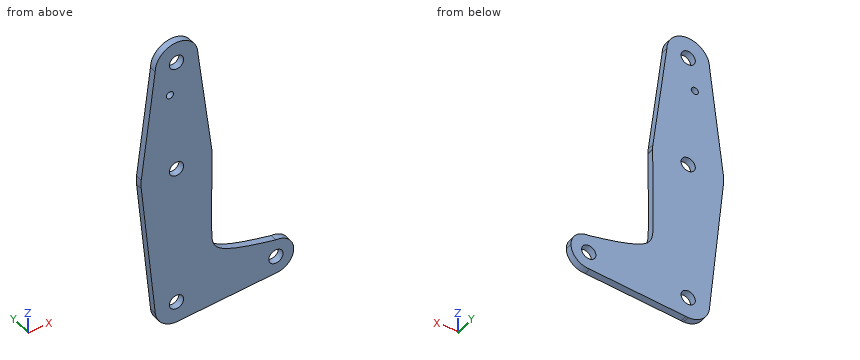
from build123d import *

# Parameters (mm, degrees)
F0_R     = 3.175
F0_R_2   = 1.5875
F1_DEPTH = 3.048


with BuildPart() as f1:
    # F0 (on Front) → F1 (new body)
    with BuildSketch(Plane.XZ):
        with BuildLine():
            add(Edge.make_bspline(
                [(15.875, 0), (15.8732372033, -0.1365743579), (15.8714744066, -0.2731487158), (15.8697119149, -0.4097178745)],
                knots=[0, 0, 0, 0, 0.0040359027, 0.0040359027, 0.0040359027, 0.0040359027], degree=3))
            ThreePointArc((15.875, 0), (15.8430821396, 1.0061676396), (15.7474569047, 2.0082893304))
            ThreePointArc((15.7474569047, 2.0082893304), (0, 15.875), (-15.7474569047, 2.0082893304))
            ThreePointArc((-15.7474569047, 2.0082893304), (-15.875, 0), (-15.7474569047, -2.0082893304))
            ThreePointArc((-15.7474569047, -2.0082893304), (0.8016197645, -15.8547478931), (15.8697119149, -0.4097178745))
        make_face()
        Circle(F0_R, mode=Mode.SUBTRACT)
        with BuildLine():
            ThreePointArc((15.8697119149, -0.4097178745), (15.8736779237, -0.2048759994), (15.875, 0))
            add(Edge.make_bspline(
                [(15.875, 0), (15.8732372033, -0.1365743579), (15.8714744066, -0.2731487158), (15.8697119149, -0.4097178745)],
                knots=[0, 0, 0, 0, 0.0040359027, 0.0040359027, 0.0040359027, 0.0040359027], degree=3))
        make_face()
        with BuildLine():
            ThreePointArc((-15.7474569047, 2.0082893304), (0, 15.875), (15.7474569047, 2.0082893304))
            Line((15.7474569047, 2.0082893304), (9.525, 50.8))
            ThreePointArc((9.525, 50.8), (0, 41.275), (-9.525, 50.8))
            Line((-9.525, 50.8), (-15.7474569047, 2.0082893304))
        make_face()
        with Locations((-2.9496776406, 36.5252)):
            Circle(F0_R_2, mode=Mode.SUBTRACT)
        with BuildLine():
            add(Edge.make_bspline(
                [(15.8697119149, -0.4097178745), (15.6873811422, -14.5378753073), (15.4159472913, -35.8693253106), (16.221504585, -48.4230919996), (33.5230137181, -52.3059412595), (44.3829082704, -54.7431467772)],
                knots=[0.0040359027, 0.0040359027, 0.0040359027, 0.0040359027, 0.421552344, 0.6369171903, 1, 1, 1, 1], degree=3))
            ThreePointArc((15.8697119149, -0.4097178745), (0.8016197645, -15.8547478931), (-15.7474569047, -2.0082893304))
            Line((-15.7474569047, -2.0082893304), (-9.4773410414, -64.4516468803))
            ThreePointArc((-9.4773410414, -64.4516468803), (-0.4764197627, -53.986922201), (9.525, -63.5))
            ThreePointArc((9.525, -63.5), (7.0949392109, -69.8551131063), (1.0446928936, -72.9675362032))
            Line((1.0446928936, -72.9675362032), (43.960813643, -70.6069159106))
            ThreePointArc((43.960813643, -70.6069159106), (36.4482164838, -62.4695247705), (44.3829082704, -54.7431467772))
        make_face()
        with BuildLine():
            ThreePointArc((-9.525, 50.8), (0, 41.275), (9.525, 50.8))
            ThreePointArc((9.525, 50.8), (0, 60.325), (-9.525, 50.8))
        make_face()
        with Locations((0, 50.8)):
            Circle(F0_R, mode=Mode.SUBTRACT)
        with BuildLine():
            ThreePointArc((52.3204082704, -62.6806467772), (49.995568346, -57.0679867015), (44.3829082704, -54.7431467772))
            ThreePointArc((44.3829082704, -54.7431467772), (36.4482164838, -62.4695247705), (43.960813643, -70.6069159106))
            ThreePointArc((43.960813643, -70.6069159106), (49.8442968367, -68.4406069487), (52.3204082704, -62.6806467772))
        make_face()
        with Locations((44.3829082704, -62.6806467772)):
            Circle(F0_R, mode=Mode.SUBTRACT)
        with BuildLine():
            ThreePointArc((9.525, -63.5), (-0.4764197627, -53.986922201), (-9.4773410414, -64.4516468803))
            ThreePointArc((-9.4773410414, -64.4516468803), (-6.3898821767, -70.5636414665), (0, -73.025))
            Line((0, -73.025), (1.0446928936, -72.9675362032))
            ThreePointArc((1.0446928936, -72.9675362032), (7.0949392109, -69.8551131063), (9.525, -63.5))
        make_face()
        with Locations((0, -63.5)):
            Circle(F0_R, mode=Mode.SUBTRACT)
        with BuildLine():
            Line((1.0446928936, -72.9675362032), (0, -73.025))
            ThreePointArc((0, -73.025), (0.5231360554, -73.0106232008), (1.0446928936, -72.9675362032))
        make_face()
    extrude(amount=F1_DEPTH)


solid = f1.part
Verification items for the finished model (mm, model axes). Coordinates: 2 decimals unless noted, no trailing zeros. Loops run counter-clockwise (first coordinate to the right, second up) from the corner with the lowest first, then second, coordinate; pieces in that order, holes last. Notation, with made-up numbers: (-13, 44) -> (32, 44) arc R23 ccw to (32, 79) -> close; hole circle Ø8 at (-31.5, 22). An arc over 180 degrees is marked (long way). Write each question's results on one line, items separated by ' | '.
Item 1: Gauge pin test, flat ends, axial feed: pin 1 (1 mm diameter, centred on x = 31, y = -2, fed in from -Z); pin 2 (1.5 mm diameter, centred on y = -2.5, z = 16, fed in from +X). Record the tip position at first contact, or that the pin passes through.
Found:
pin 1: stops at z = -71.35 | pin 2: stops at x = 14.06
Item 2: Section check B-B, the plane z = 10. Enter the section's corners in (x, y).
Found:
outline: (-14.73, -3.05) -> (14.73, -3.05) -> (14.73, 0) -> (-14.73, 0) -> close
Item 3: Material ranges on L1, parallel to X at y = -0.65, z = 53; L2, parallel to Z at x = 43, y = -0.6; L3, parallel to Z at x = 43.5, y = -2, recorded low to high.
Found:
L1: x = -9.27 to -2.29, 2.29 to 9.27 | L2: z = -70.66 to -65.54, -59.82 to -54.43 | L3: z = -70.63 to -65.73, -59.63 to -54.54
Item 4: Section check A-A, the plane y = -1.1. Count the separate pieces of the cut face and the enclosed holes in it, plus the area to 3 significant figures.
Found:
separate pieces: 1 | enclosed holes: 5 | area: 4,020 mm2
